The figure shows three views and two pictorial views of one solid part (mm, origin at its lowest corner). Answer the questions. A direction names the side the tool comes from. Round coordinates to 2 decimals unless told otherwise and drop trailing zeros. Order: outer loops, then holes, each group sorted by start corner. A loop starts at its lowest first (then second) coordinate and runs counter-clockwise, first axis right, second up. Notation, with made-up numbers: (81, 26) - (110, 26) arc R27 ccw to (110, 47) - close; hole circle Ø5 at (67.5, 41.5). An arc over 180 degrees is marked (long way). Answer as a JSON object with one key per item and string values. Group by question number.
Q1. A cutting plane is placed at B-B on z = 3.75. Determine the outline of the cut face in (x, y), and give its area (3 significant figures).
Q2. The mould has two halves that part along X. Classify the marked faces 1, 2 and 3: pulls with the +X half, pulls with the -X half, needs draft (parallel to the pull), parting line crosses it, or undercut.
Q3. Consider line 1 (Y direction, x = 25, z = 1.65); line 2 (X direction, y = 33, z = 9) (1 decimal); line 3 (X direction, y = 30, z = 9.25) (1 decimal). Determine where each line is inside the solid, lowest interval first.
Q4. A cutting plane is placed at C-C on x = 12. Determine the outline of the cut face in (y, z) (1 decimal).
Q5. A cutting plane is placed at D-D on x = 68. Determine the outline of the cut face in (y, z), and give its area (3 significant figures).
Q6. A cutting plane is placed at A-A on y = 9. Determine the outline of the cut face in (x, z), and give its area (3 significant figures).
Q7. Given pin 1 Ø1.5 at (x, z) = (76.5, 8) entering from +Y; pin 2 Ø1.5 at (y, z) = (14, 18.5) entering from -X; pin 3 Ø10 at (y, z) = (38.5, 18) entering from -X, each flat-ended and moving along its own axis, determine where each tip first touches the part or whether it passes through.
Q8. A tool of negligible diameter and unlimited length cuts with its end or side. For the marked faces 4, 5 and 6, from which of +Z, -Z, +X, -X, +Y, -Y can it reach the whole face along a straight path? Write none if from no direction.
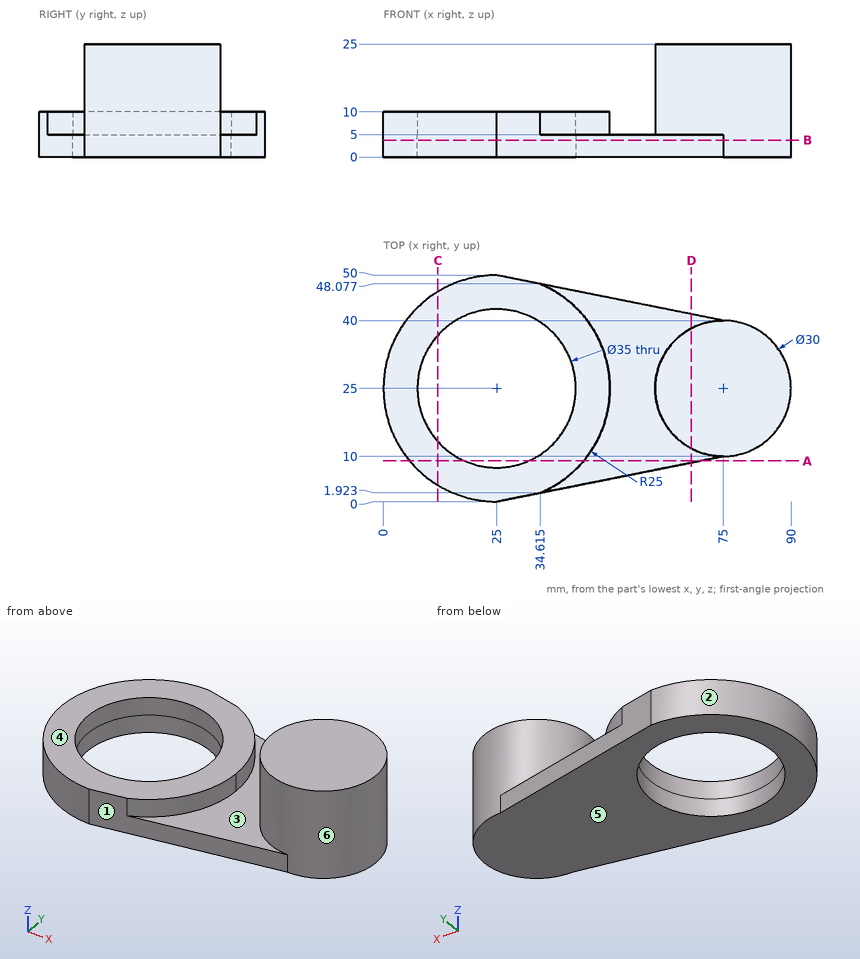
Result set:
{
 "1": {"outline": "(25, 0) - (75, 10) arc R15 ccw to (75, 40) - (25, 50) arc R25 ccw to start; hole circle Ø35 at (25, 25)", "area": "2,370 mm²"},
 "2": {"face 1": "pulls with the +X half", "face 2": "pulls with the -X half", "face 3": "undercut"},
 "3": {"line 1": "y = 0 to 7.5, 42.5 to 50", "line 2": "x = 1.3 to 9.4, 40.6 to 48.7, 62.3 to 87.7", "line 3": "x = 0.5 to 8.2, 41.8 to 49.5, 60.9 to 89.1"},
 "4": {"outline": "(3.6, 0) - (13.3, 0) - (13.3, 10) - (3.6, 10) - close; (36.7, 0) - (46.4, 0) - (46.4, 10) - (36.7, 10) - close"},
 "5": {"outline": "(8.6, 0) - (41.4, 0) - (41.4, 5) - (38.27, 5) - (38.27, 25) - (11.73, 25) - (11.73, 5) - (8.6, 5) - close", "area": "695 mm²"},
 "6": {"outline": "(5.79, 0) - (17.91, 0) - (17.91, 10) - (5.79, 10) - close; (32.09, 0) - (70, 0) - (70, 5) - (44.21, 5) - (44.21, 10) - (32.09, 10) - close", "area": "371 mm²"},
 "7": {"pin 1": "stops at y = 39.98", "pin 2": "stops at x = 64.05", "pin 3": "stops at x = 62.64"},
 "8": {"face 4": "+Z, -X, +Y, -Y", "face 5": "-Z, +X, -X, +Y, -Y", "face 6": "+Z"}
}
